The model under review builds one solid part; all positions refer to its coordinate system, in mm. Face numbers are marked on the shaded views. A direction names the side the tool comes from. Give positions to 0.01 mm unless a question says otherwise; leave off trailing zeros. Write each loop counter-clockwise with the first axis right and the second up, starting at its lowest first coordinate (ties: lowest second). Pieces come first, ordered by that corner, then holes. Notation, with made-up numbers: M 6.25,-4.5 L 61.25,-4.5 A23 ccw 61.25,33.5 Z; hole C 86.5,65.5 d11. An arc over 180 degrees is marked long. Write each question's results on one line, items separated by ' | '. Start each with the question number.
Autodesk Inventor part; units mm, degrees
ref_plane "Work Plane1" through (40, 0, 0) normal (1, 0, 0) x (0, 0, -1)
ref_plane "YZ Plane" through (0, 0, 0) normal (1, 0, 0) x (0, 1, 0)
ref_plane "XZ Plane" through (0, 0, 0) normal (0, 1, 0) x (-1, 0, 0)
sketch "Sketch1" plane through (0, 0, 0) normal (1, 0, 0) x (0, 1, 0)
  line L0 (-10, 35) -> (10, 35)
  line L1 (10, 35) -> (10, -35)
  line L2 (10, -35) -> (-10, -35)
  line L3 (-10, -35) -> (-10, 35)
  line L4 (-10, 35) -> (10, -35) construction
  line L5 (10, 35) -> (-10, -35) construction
  point P0 (0, 0)
  dimension "d0" = 20
  dimension "d1" = 70
extrude "Extrusion1" add sketch "Sketch1" along normal blind 80
sketch "Sketch2" plane through (80, 0, 0) normal (1, 0, 0) x (0, 0, -1)
  line L0 (-35, 10) -> (-35, -10)
  line L1 (-35, 0) -> (35, 0)
  line L2 (35, -10) -> (35, 10)
  line L3 (35, 10) -> (-35, 10)
  line L4 (0, 10) -> (0, -10)
  line L5 (-35, -10) -> (35, -10)
  point P0 (0, 0)
  point P1 (-25, 0)
  point P2 (25, 0)
  dimension "d4" = 25
hole "Hole1" at (80, 0, 25) at (80, 0, -25) direction (-1, 0, 0) diameter 10.106 depth 24 tip angle 118
ref_plane "Work Plane1" through (40, 0, 0) normal (1, 0, 0) x (0, 0, -1)
mirror "Mirror1" about plane through (40, 0, 0) normal (1, 0, 0) of "Hole1"
fillet "Fillet1" radius 2 4 edges at (40, 10, 35) (40, -10, 35) (40, -10, -35) (40, 10, -35)
sketch "Sketch3" plane through (0, 10, 33) normal (0, 1, 0) x (1, 0, 0)
  line L0 (80, 0) -> (80, 66)
  line L1 (80, 33) -> (0, 33)
  point P0 (40, 33)
hole "Hole2" at (40, 10, 0) direction (0, -1, 0) diameter 6.647 end through all
properties part number "Profile_Middle_03"
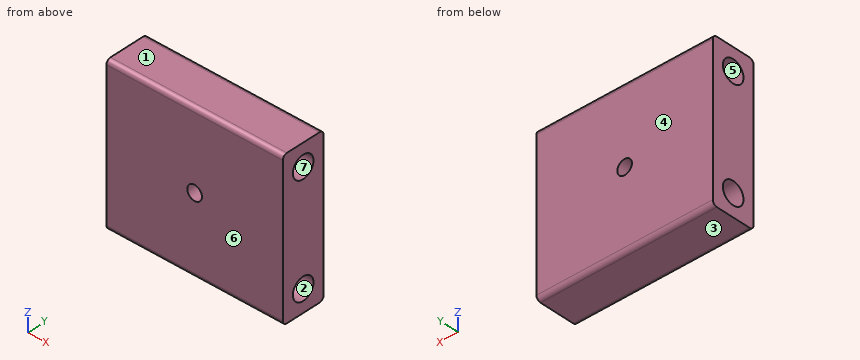
(1) Clearance check with flat-ended pins moving along their axes: P1, Ø10, axis at y = -6, z = 5.5, coming from the -X side; P2, Ø9, axis at y = 0, z = -25, coming from the -X side; P3, Ø9, axis at y = 0, z = 25, coming from the +X side. State where each tip first meets the part, or that it passes through.
(2) Draft analysis for pull direction Z (two halves, no side actions). For the marked faces 1, 2, 3 and 4, state which applies: pulls with the +Z half, pulls with the -Z half, needs draft (parallel to the pull), parting line crosses it, or undercut.
(3) Add section A-A (x = 22.5). State the section outline as (y, z) points, then the cut area to 3 significant figures.
(4) Wall thickness on L1, parallel to Z at x = 71.25, y = 0; L2, parallel to Y at x = 6.5, z = -25; L3, parallel to X at y = -5.75, z = 0: over which ranges is each line inside the solid? List them lowest first.
(5) Add section B-B (x = 40). State the section outline as (y, z) points.
(6) Machinability: for the marked faces 5, 6 and 7, which of the approach directions +Z, -Z, +X, -X, +Y, -Y give a long, thin tool a straight path to every point of the face, cutting with its end or side? Answer none if there is none.
Calculated:
1) P1: stops at x = 0 | P2: stops at x = 24.33 | P3: stops at x = 55.67
2) face 1: pulls with the +Z half | face 2: undercut | face 3: pulls with the -Z half | face 4: needs draft
3) outline: M -10,-33 A2 ccw -8,-35 L 8,-35 A2 ccw 10,-33 L 10,33 A2 ccw 8,35 L -8,35 A2 ccw -10,33 Z; hole C 0,-25 d10.11; hole C 0,25 d10.11 | area: 1,240 mm²
4) L1: z = -35 to -30.05, -19.95 to 19.95, 30.05 to 35 | L2: y = -10 to -5.05, 5.05 to 10 | L3: x = 0 to 36.68, 43.32 to 80
5) outline: M -10,-33 A2 ccw -8,-35 L 8,-35 A2 ccw 10,-33 L 10,-3.32 L -10,-3.32 Z; M -10,3.32 L 10,3.32 L 10,33 A2 ccw 8,35 L -8,35 A2 ccw -10,33 Z
6) face 5: -X | face 6: +Z, -Z, +X, -X, -Y | face 7: +X
